from build123d import *

# Parameters (mm, degrees)
BOSS_EXTRUDE1_DEPTH = 2
SKETCH1_3_R         = 2.75
SKETCH1_3_R_2       = 1.75
BOSS_EXTRUDE2_DEPTH = 4.5


with BuildPart() as part:
    # Sketch1 → Boss-Extrude1 (new body)
    with BuildSketch(Plane.XY):
        with BuildLine():
            Line((4, -16), (4, 0))
            ThreePointArc((4, 0), (0, 4), (-4, 0))
            Line((-4, 0), (-4, -16))
            ThreePointArc((-4, -16), (0, -20), (4, -16))
        make_face()
    extrude(amount=-BOSS_EXTRUDE1_DEPTH)

    # Sketch1<3> → Boss-Extrude2 (add)
    # profile 1 of 2: a face of its own
    with BuildSketch(Plane.XY):
        Circle(SKETCH1_3_R)
        Circle(SKETCH1_3_R_2, mode=Mode.SUBTRACT)
    # profile 2 of 2: a face of its own
    with BuildSketch(Plane.XY):
        with Locations((0, -16)):
            Circle(SKETCH1_3_R)
        with Locations((0, -16)):
            Circle(SKETCH1_3_R_2, mode=Mode.SUBTRACT)
    extrude(amount=BOSS_EXTRUDE2_DEPTH)


solid = part.part
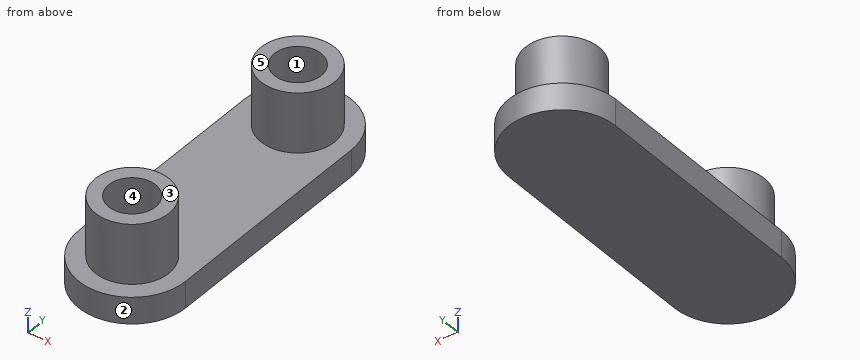
Can you work these out from the model? Positions are in its coordinate system, mm. Face numbers are marked on the shaded views. A direction names the side the tool comes from. Coordinates: 2 decimals unless noted, no trailing zeros. Loops run counter-clockwise (first coordinate to the right, second up) from the corner with the lowest first, then second, coordinate; pieces in that order, holes last. Notation, with made-up numbers: (86, 81) - (118, 81) arc R15 cw to (118, 103) - close; hole circle Ø3 at (-20, 25). An arc over 180 degrees is marked (long way). Answer as a JSON object with one key per item and string values. Group by question number.
Item 1: If we section it at A-A (z = 0.75): List the corners of the cut face in (x, y) for me, plus the area to 3 significant figures.
Item 2: If we section it at B-B (x = 0): List the corners of the cut face in (y, z) for me.
Item 3: For pin 1 (1.8 mm diameter, centred on x = 0.5, y = -15.5, fed in from +Z); pin 2 (2 mm diameter, centred on y = -14, z = 2, fed in from -X); pin 3 (2 mm diameter, centred on x = -2.5, z = -0.5, fed in from +Y), each with a flat end and sliding along its axis, tell me the tip position at first contact or that it passes through.
Item 4: On a 3-axis mill with a long thin cutter (end or side, diameter ignored), from which of +Z, -Z, +X, -X, +Y, -Y can I reach the whole of each face in a straight line? I mean the marked faces 4 and 5. Say none if no direction works.
Item 5: If we mould it in two halves opening along Y, with no side actions, what happens to the marked faces 1, 2 and 3? For each: released by +Y, released by -Y, zero draft, split by the parting line, or undercut.
Item 6: If we section it at D-D (z = -1.25): List the corners of the cut face in (x, y) for me.
Item 7: If we section it at C-C (y = -6.75): List the corners of the cut face in (x, z) for me, plus the area to 3 significant figures.
Item 8: If I drill on L1, parallel to Y at x = 0, z = 2; L2, parallel to Z at x = -2, y = -2.25; L3, parallel to Y at x = 1.25, z = 1.5, over which ranges is the centre line in solid material (lowest first)? Write a range as from..to.
Returned:
{
 "1": {"outline": "circle Ø5.5 at (0, -16); circle Ø5.5 at (0, 0); hole circle Ø3.5 at (0, -16); hole circle Ø3.5 at (0, 0)", "area": "28.3 mm²"},
 "2": {"outline": "(-20, -2) - (4, -2) - (4, 0) - (2.75, 0) - (2.75, 4.5) - (1.75, 4.5) - (1.75, 0) - (-1.75, 0) - (-1.75, 4.5) - (-2.75, 4.5) - (-2.75, 0) - (-13.25, 0) - (-13.25, 4.5) - (-14.25, 4.5) - (-14.25, 0) - (-17.75, 0) - (-17.75, 4.5) - (-18.75, 4.5) - (-18.75, 0) - (-20, 0) - close"},
 "3": {"pin 1": "stops at z = 0", "pin 2": "stops at x = -2.56", "pin 3": "stops at y = 3.71"},
 "4": {"face 4": "+Z", "face 5": "+Z, +X, -X, +Y, -Y"},
 "5": {"face 1": "undercut", "face 2": "released by -Y", "face 3": "zero draft"},
 "6": {"outline": "(-4, -16) arc R4 ccw to (4, -16) - (4, 0) arc R4 ccw to (-4, 0) - close"},
 "7": {"outline": "(-4, -2) - (4, -2) - (4, 0) - (-4, 0) - close", "area": "16.0 mm²"},
 "8": {"L1": "y = -18.75..-17.75, -14.25..-13.25, -2.75..-1.75, 1.75..2.75", "L2": "z = -2..0", "L3": "y = -18.45..-17.22, -14.78..-13.55, -2.45..-1.22, 1.22..2.45"}
}
